Model file for the job. Use its own axes, mm. Face numbers are marked on the shaded views. A direction names the side the tool comes from. Round coordinates to 2 decimals unless told otherwise and drop trailing zeros. Loops run counter-clockwise (first coordinate to the right, second up) from the corner with the lowest first, then second, coordinate; pieces in that order, holes last. Notation, with made-up numbers: (61, -37) -> (106, -37) arc R21 cw to (106, -11) -> close; hole circle Ø6 at (-18.5, 73.5). An arc over 180 degrees is marked (long way). Use a Markdown table: item, result.
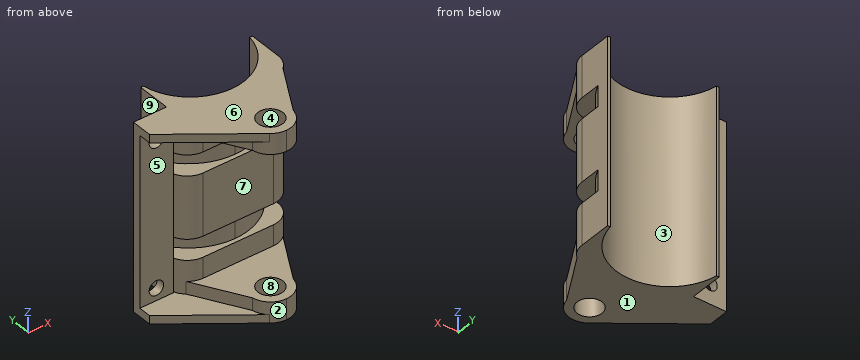
from build123d import *

# Parameters (mm, degrees)
BOSS_EXTRUDE1_DEPTH = 45
SKETCH2_W           = 10
SKETCH2_H           = 5
BOSS_EXTRUDE2_DEPTH = 15
SKETCH3_R           = 3
CUT_EXTRUDE1_DEPTH  = 50.317846668
FILLET1_R           = 5
CUT_EXTRUDE2_DEPTH  = 5
LPATTERN1_COUNT     = 2
LPATTERN1_PITCH     = 20
CHAMFER1_DEPTH      = 5
CHAMFER1_START      = 40
CHAMFER1_2_DEPTH    = 5
BOSS_EXTRUDE3_DEPTH = 2
BOSS_EXTRUDE9_REACH = 52.361
SKETCH8_W           = 8.2
SKETCH8_H           = 2
SKETCH9_R           = 1.75
CUT_EXTRUDE4_DEPTH  = 47


with BuildPart() as part:
    # Sketch1 → Boss-Extrude1 (new body)
    with BuildSketch(Plane.XY):
        with BuildLine():
            Line((12.845232579, 13), (13.5, 13))
            Line((13.5, 13), (13.5, 5))
            ThreePointArc((13.5, 5), (12.035533906, 1.464466094), (8.5, 0))
            Line((8.5, 0), (-8.5, 0))
            ThreePointArc((-8.5, 0), (-12.035533906, 1.464466094), (-13.5, 5))
            Line((-13.5, 5), (-13.5, 13))
            Line((-13.5, 13), (-12.845232579, 13))
            ThreePointArc((-12.845232579, 13), (0, 2), (12.845232579, 13))
        make_face()
    extrude(amount=BOSS_EXTRUDE1_DEPTH)

    # Sketch2 → Boss-Extrude2 (add)
    with BuildSketch(Plane.XZ):
        with Locations((0, 42.5)):
            Rectangle(SKETCH2_W, SKETCH2_H)
        with Locations((0, 2.5)):
            Rectangle(SKETCH2_W, SKETCH2_H)
    extrude(amount=BOSS_EXTRUDE2_DEPTH)

    # Sketch3 → Cut-Extrude1 (cut, through all)
    with BuildSketch(Plane.XY.offset(45)):
        with Locations((0, -10)):
            Circle(SKETCH3_R)
    extrude(amount=-CUT_EXTRUDE1_DEPTH, mode=Mode.SUBTRACT)

    # Fillet1
    fillet1_edges = [part.edges().sort_by_distance(p)[0] for p in [
        (-5, -15, 2.5),
        (-5, -15, 42.5),
        (5, -15, 42.5),
        (5, -15, 2.5),
    ]]
    fillet(fillet1_edges, radius=FILLET1_R - 0.0001)  # a hair under: the kernel refuses the full size

    # Sketch4 → Cut-Extrude2 (cut)
    with BuildSketch(Plane.XY.offset(10)):
        with BuildLine():
            Line((-13.5, 10), (-13.5, 5))
            ThreePointArc((-13.5, 5), (-12.035533906, 1.464466094), (-8.5, 0))
            Line((-8.5, 0), (5, 0))
            Line((5, 0), (8.5, 0))
            ThreePointArc((8.5, 0), (12.035533906, 1.464466094), (13.5, 5))
            Line((13.5, 5), (13.5, 10))
            ThreePointArc((13.5, 10), (8.11249037, 3.456264445), (0, 1))
            ThreePointArc((0, 1), (-8.11249037, 3.456264445), (-13.5, 10))
        make_face()
    cut_extrude2 = extrude(amount=CUT_EXTRUDE2_DEPTH, mode=Mode.SUBTRACT)

    # LPattern1: Cut-Extrude2 ×2
    with Locations(*[(0, 0, i * LPATTERN1_PITCH) for i in range(1, LPATTERN1_COUNT)]):
        add(cut_extrude2, mode=Mode.SUBTRACT)

    # Chamfer1: read off the stored shape, not the designer's step
    # Chamfer1 outline → Chamfer1 (add)
    with BuildSketch(Plane.XY):
        with BuildLine():
            ThreePointArc((5, -10), (4.983300978, -10.408303031), (4.933315454, -10.813878757))
            Line((4.933315454, -10.813878757), (11.733315454, 1.186121243))
            ThreePointArc((11.733315454, 1.186121243), (10.222005548, 0.305886996), (8.5, 0))
            Line((8.5, 0), (5, 0))
            Line((5, 0), (5, -10))
        make_face()
        with BuildLine():
            Line((-11.733315454, 1.186121243), (-4.933315454, -10.813878757))
            ThreePointArc((-4.933315454, -10.813878757), (-4.983300978, -10.408303031), (-5, -10))
            Line((-5, -10), (-5, 0))
            Line((-5, 0), (-8.5, 0))
            ThreePointArc((-8.5, 0), (-10.222005548, 0.305886996), (-11.733315454, 1.186121243))
        make_face()
    extrude(amount=CHAMFER1_DEPTH)

    # Chamfer1 2 outline → Chamfer1 2 (add)
    with BuildSketch(Plane.XY.offset(CHAMFER1_START)):
        with BuildLine():
            ThreePointArc((5, -10), (4.983300978, -10.408303031), (4.933315454, -10.813878757))
            Line((4.933315454, -10.813878757), (11.733315454, 1.186121243))
            ThreePointArc((11.733315454, 1.186121243), (10.222005548, 0.305886996), (8.5, 0))
            Line((8.5, 0), (5, 0))
            Line((5, 0), (5, -10))
        make_face()
        with BuildLine():
            Line((-11.733315454, 1.186121243), (-4.933315454, -10.813878757))
            ThreePointArc((-4.933315454, -10.813878757), (-4.983300978, -10.408303031), (-5, -10))
            Line((-5, -10), (-5, 0))
            Line((-5, 0), (-8.5, 0))
            ThreePointArc((-8.5, 0), (-10.222005548, 0.305886996), (-11.733315454, 1.186121243))
        make_face()
    extrude(amount=CHAMFER1_2_DEPTH)

    # Sketch6 → Boss-Extrude3 (add)
    with BuildSketch(Plane(origin=(0, 0, 0), x_dir=(-1, 0, 0), z_dir=(0, 0, -1))):
        Polygon((3.223775495, -13.830713979), (21.5, 0), (21.5, 5), (13.5, 5), align=None)
    boss_extrude3 = extrude(amount=-BOSS_EXTRUDE3_DEPTH)

    # Mirror1: Boss-Extrude3 across plane
    add(boss_extrude3.mirror(Plane.XY.offset(22.5)))

    # Sketch8 → Boss-Extrude9 (add, up to next)
    with BuildSketch(Plane.XY.offset(2), mode=Mode.PRIVATE) as boss_extrude9_sk1:
        with Locations((-17.4, 4)):
            Rectangle(SKETCH8_W, SKETCH8_H)
    boss_extrude9_tool1 = extrude(boss_extrude9_sk1.sketch, amount=BOSS_EXTRUDE9_REACH, mode=Mode.PRIVATE) - part.part
    add(boss_extrude9_tool1.solids().sort_by_distance((-17.4, 4, 2))[0])

    # Sketch9 → Cut-Extrude4 (cut)
    with BuildSketch(Plane(origin=(0, 5, 0), x_dir=(1, 0, 0), z_dir=(0, 1, 0))):
        with Locations(Location((-17.5, -5, 0), (0, 0, 180))):
            Circle(SKETCH9_R)
        with Locations(Location((-17.5, -40, 0), (0, 0, 180))):
            Circle(SKETCH9_R)
    extrude(amount=-CUT_EXTRUDE4_DEPTH, mode=Mode.SUBTRACT)


solid = part.part
Q1. Tool access for the marked faces 5, 6, 7, 8 and 9: list every direction of +Z, -Z, +X, -X, +Y, -Y with a clear straight run to the whole face (end or side of a thin tool).
Results list:
| item | result |
|---|---|
| face 5 | -X, -Y |
| face 6 | +Z, +X, -X, +Y, -Y |
| face 7 | +X, -X, -Y |
| face 8 | +Z, -Z |
| face 9 | +Z, -Z, -X, +Y |
Q2. Pull direction X, two halves, no side cores. Call the marked faces 1, 2, 3 and 4: released by +X, released by -X, zero draft, split by the parting line, or undercut.
Results list:
| item | result |
|---|---|
| face 1 | zero draft |
| face 2 | released by -X |
| face 3 | undercut |
| face 4 | undercut |
Q3. Band-saw the part on B-B, the plane y = -10. Give the cut face in (x, z), plus the area to 3 significant figures.
Results list:
| item | result |
|---|---|
| outline | (-8.29, 0) -> (-3, 0) -> (-3, 5) -> (-5.39, 5) -> (-5.39, 2) -> (-8.29, 2) -> close; (-8.29, 43) -> (-5.39, 43) -> (-5.39, 40) -> (-3, 40) -> (-3, 45) -> (-8.29, 45) -> close; (3, 0) -> (5.39, 0) -> (5.39, 5) -> (3, 5) -> close; (3, 40) -> (5.39, 40) -> (5.39, 45) -> (3, 45) -> close |
| area | 59.5 mm² |
Q4. Band-saw the part on A-A, the plane x = -17.5. Give the cut face in (y, z), plus the area to 3 significant figures.
Results list:
| item | result |
|---|---|
| outline | (-3.03, 0) -> (5, 0) -> (5, 3.25) -> (3, 3.25) -> (3, 2) -> (-3.03, 2) -> close; (-3.03, 43) -> (3, 43) -> (3, 41.75) -> (5, 41.75) -> (5, 45) -> (-3.03, 45) -> close; (3, 6.75) -> (5, 6.75) -> (5, 38.25) -> (3, 38.25) -> close |
| area | 100 mm² |
Q5. Flat gauge pins, fed straight in: pin 1 (4.5 mm diameter, centred on x = -4, z = 23.5, fed in from -Y); pin 2 (6.5 mm diameter, centred on y = 10.5, z = 30.5, fed in from -X); pin 3 (3 mm diameter, centred on x = -6.5, y = 6.5, fed in from -Z); pin 4 (4 mm diameter, centred on x = -16.5, z = 14.5, fed in from +Y). Where does each tip first touch, or does it go through?
Results list:
| item | result |
|---|---|
| pin 1 | stops at y = 0 |
| pin 2 | stops at x = -13.5 |
| pin 3 | passes through |
| pin 4 | stops at y = 5 |
Q6. Drill centre lines: L1, parallel to Z at x = -17.5, y = 4.5; L2, parallel to Z at x = -11.5, y = -0.5; L3, parallel to Z at x = -3.5, y = -8. Where is each one in solid material? Low to high. Write a range as from..to.
Results list:
| item | result |
|---|---|
| L1 | z = 0..3.25, 6.75..38.25, 41.75..45 |
| L2 | z = 0..2, 43..45 |
| L3 | z = 0..5, 40..45 |
Q7. Band-saw the part on C-C, the plane z = 29. Give the cut face in (x, y), plus the area to 3 significant figures.
Results list:
| item | result |
|---|---|
| outline | (-21.5, 3) -> (-13.3, 3) -> (-13.3, 3.6) arc R5 ccw to (-8.5, 0) -> (8.5, 0) arc R5 ccw to (13.5, 5) -> (13.5, 13) -> (12.85, 13) arc R13 cw to (-12.85, 13) -> (-13.5, 13) -> (-13.5, 5) -> (-21.5, 5) -> close |
| area | 143 mm² |
Q8. Band-saw the part on D-D, the plane y = 9. Give the cut face in (x, z), plus the area to 3 significant figures.
Results list:
| item | result |
|---|---|
| outline | (-13.5, 0) -> (-11.53, 0) -> (-11.53, 45) -> (-13.5, 45) -> (-13.5, 35) -> (-13.04, 35) -> (-13.04, 30) -> (-13.5, 30) -> (-13.5, 15) -> (-13.04, 15) -> (-13.04, 10) -> (-13.5, 10) -> close; (11.53, 0) -> (13.5, 0) -> (13.5, 10) -> (13.04, 10) -> (13.04, 15) -> (13.5, 15) -> (13.5, 30) -> (13.04, 30) -> (13.04, 35) -> (13.5, 35) -> (13.5, 45) -> (11.53, 45) -> close |
| area | 168 mm² |
